Geometry check sheet. Reference: the model listing, model coordinates, mm. Round coordinates to 2 decimals unless told otherwise and drop trailing zeros. Order: outer loops, then holes, each group sorted by start corner. A loop starts at its lowest first (then second) coordinate and runs counter-clockwise, first axis right, second up.
```python
from build123d import *

# Parameters (mm, degrees)
F0_R            = 11
F1_DEPTH        = 2
F2_W            = 3
F2_H            = 1.5
F3_DEPTH        = 2
F3_COPIES_COUNT = 20
F4_R            = 4
F5_DEPTH        = 4
F5_DEPTH_BACK   = 4
F7_DEPTH        = 9


# Not quite as in the source:
# - a pattern or mirror of a feature is missing from the dataset's text; its kind, count and spacing are read off the source's solid


with BuildPart() as f1:
    # F0 (on Top) → F1 (new body)
    with BuildSketch(Plane.XY):
        Circle(F0_R)
    extrude(amount=F1_DEPTH)

    # F2 (on face) → F3 (cut)
    with BuildSketch(Plane.XY.offset(2)):
        with Locations((8.5, 0)):
            Rectangle(F2_W, F2_H)
    f3 = extrude(amount=-F3_DEPTH, mode=Mode.SUBTRACT)

    # F3_copies: F3 ×20 about axis
    f3_copies_axis = Axis((0, 0, 0), (0, 0, 1))
    for i in range(1, F3_COPIES_COUNT):
        add(f3.rotate(f3_copies_axis, i * 360 / F3_COPIES_COUNT), mode=Mode.SUBTRACT)

    # F4 (on face) → F5 (join, two sides)
    with BuildSketch(Plane(origin=(0, 0, 0), x_dir=(1, 0, 0), z_dir=(0, 0, -1))) as f5_sk:
        Circle(F4_R)
    extrude(amount=F5_DEPTH)
    extrude(f5_sk.sketch, amount=-F5_DEPTH_BACK)

    # F6 (on face) → F7 (cut)
    with BuildSketch(Plane.XY.offset(4)):
        with BuildLine():
            Line((-2.3048861143, -1.5), (2.3048861143, -1.5))
            ThreePointArc((2.3048861143, -1.5), (2.75, 0), (2.3048861143, 1.5))
            Line((2.3048861143, 1.5), (-2.3048861143, 1.5))
            ThreePointArc((-2.3048861143, 1.5), (-2.75, 0), (-2.3048861143, -1.5))
        make_face()
    extrude(amount=-F7_DEPTH, mode=Mode.SUBTRACT)


solid = f1.part
```
(1) Sectioned sample at D-D, the plane z = 3.25. Record the cut outline in (x, y), and give its area (3 significant figures).
Returned:
outline: circle Ø8 at (0, 0); hole (-2.3, -1.5) - (2.3, -1.5) arc R2.75 ccw to (2.3, 1.5) - (-2.3, 1.5) arc R2.75 ccw to start
area: 34.6 mm2
(2) Sectioned sample at A-A, the plane x = 0. Record the cut outline in (y, z).
Returned:
outline: (-11, 0) - (-10, 0) - (-10, 2) - (-11, 2) - close; (-7, 0) - (-4, 0) - (-4, -4) - (-1.5, -4) - (-1.5, 4) - (-4, 4) - (-4, 2) - (-7, 2) - close; (1.5, -4) - (4, -4) - (4, 0) - (7, 0) - (7, 2) - (4, 2) - (4, 4) - (1.5, 4) - close; (10, 0) - (11, 0) - (11, 2) - (10, 2) - close
(3) Material ranges on line 1 (X direction, y = 7.5, z = 1.5); line 2 (Y direction, x = -8.25, z = 1.5); line 3 (X direction, y = 1, z = -2.25), recorded low to high.
Returned:
line 1: x = -8.05 to -6.38, -4.52 to -3.23, -1.65 to -0.75, 0.75 to 1.65, 3.23 to 4.52, 6.38 to 8.05
line 2: y = -7.28 to -5.66, -5.07 to -3.47, -1.89 to -0.75, 0.75 to 1.89, 3.47 to 5.07, 5.66 to 7.28
line 3: x = -3.87 to -2.56, 2.56 to 3.87
(4) Sectioned sample at B-B, the plane y = 0. Record the cut outline in (x, z).
Returned:
outline: (-11, 0) - (-10, 0) - (-10, 2) - (-11, 2) - close; (-7, 0) - (-4, 0) - (-4, -4) - (-2.75, -4) - (-2.75, 4) - (-4, 4) - (-4, 2) - (-7, 2) - close; (2.75, -4) - (4, -4) - (4, 0) - (7, 0) - (7, 2) - (4, 2) - (4, 4) - (2.75, 4) - close; (10, 0) - (11, 0) - (11, 2) - (10, 2) - close
(5) Draft check along Y on faces 1 (the flat face through (0, 1.5, 0)), 2 (the cylindrical face through (-2.38, -10.74, 0.99)), 3 (the flat face through (5, 0, 0)). Enter one of: released by +Y, released by -Y, zero draft, split by the parting line, or undercut.
Returned:
face 1: undercut
face 2: split by the parting line
face 3: zero draft
(6) Depth check by flat-ended pin: P1, Ø1.6, axis at x = 0.5, z = 0.5, coming from the -Y side; P2, Ø1, axis at y = 8.5, z = 0.5, coming from the +X side; P3, Ø2, axis at x = -8.5, z = 0.5, coming from the -Y side; P4, Ø0.6, axis at x = 8, z = 1, coming from the -Y side. Enter the tip coordinate at first touch or a pass-through.
Returned:
P1: stops at y = -11
P2: stops at x = 7.55
P3: stops at y = -8.05
P4: stops at y = -7.86
(7) Sectioned sample at C-C, the plane x = 8.25. Record the cut outline in (y, z).
Returned:
outline: (-7.28, 0) - (-5.66, 0) - (-5.66, 2) - (-7.28, 2) - close; (-5.07, 0) - (-3.47, 0) - (-3.47, 2) - (-5.07, 2) - close; (-1.89, 0) - (-0.75, 0) - (-0.75, 2) - (-1.89, 2) - close; (0.75, 0) - (1.89, 0) - (1.89, 2) - (0.75, 2) - close; (3.47, 0) - (5.07, 0) - (5.07, 2) - (3.47, 2) - close; (5.66, 0) - (7.28, 0) - (7.28, 2) - (5.66, 2) - close
